Can you work these out from the drawing? Everything is in mm from the part's minimum corner. Coordinates: 2 decimals unless noted, no trailing zeros. Write each loop counter-clockwise with the first axis right and the second up, starting at its lowest first coordinate (ties: lowest second). Pieces come first, ordered by that corner, then holes. Notation, with made-up numbers: M -35.5,66 L 21.5,66 A20 ccw 21.5,86 Z; hole C 26,-18 d5. An arc over 180 degrees is marked long. Write item = value, one per line.
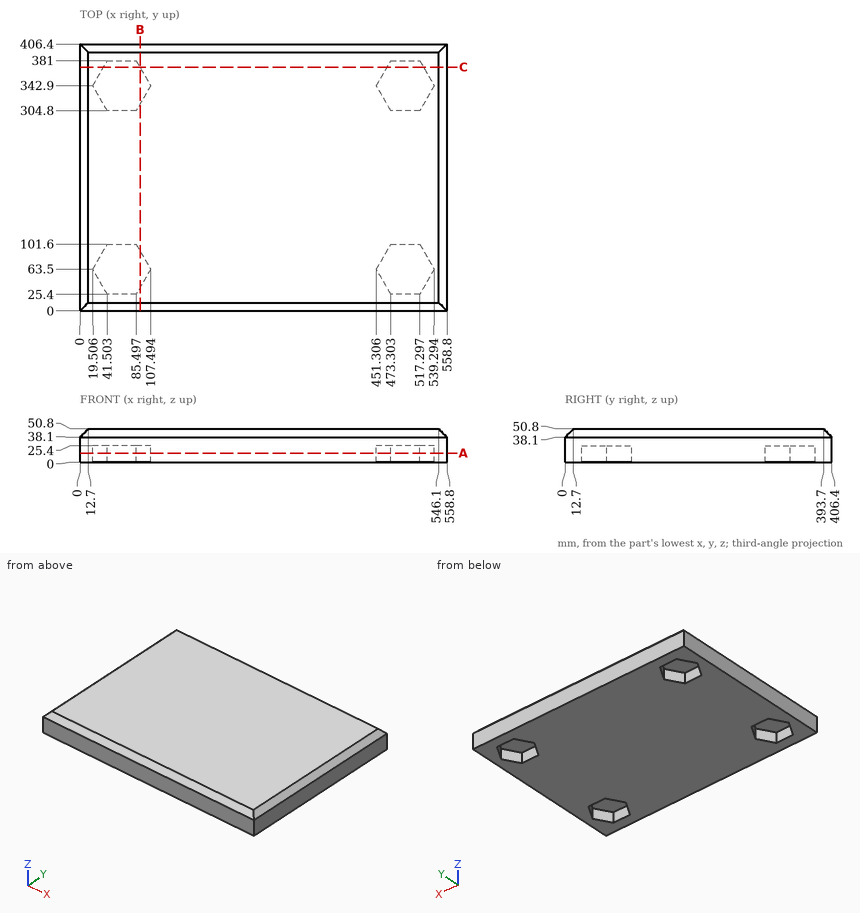
Item 1: If I drill on line 1 along Y through (x, z) = (71, 19); line 2 along X through (y, z) = (354, 6); line 3 along X through (y, z) = (77.5, 10), over which ranges is the centre line in solid material (lowest first)?
Numbers:
line_1 = 0 to 25.4, 101.6 to 304.8, 381 to 406.4
line_2 = 0 to 25.91, 101.09 to 457.71, 532.89 to 558.8
line_3 = 0 to 27.59, 99.41 to 459.39, 531.21 to 558.8
Item 2: Imagine slicing it at A-A (z = 14). Write out the boundary of the cut face in (x, y).
Numbers:
outline = M 0,0 L 558.8,0 L 558.8,406.4 L 0,406.4 Z; hole M 19.51,63.5 L 41.5,25.4 L 85.5,25.4 L 107.49,63.5 L 85.5,101.6 L 41.5,101.6 Z; hole M 19.51,342.9 L 41.5,304.8 L 85.5,304.8 L 107.49,342.9 L 85.5,381 L 41.5,381 Z; hole M 451.31,63.5 L 473.3,25.4 L 517.3,25.4 L 539.29,63.5 L 517.3,101.6 L 473.3,101.6 Z; hole M 451.31,342.9 L 473.3,304.8 L 517.3,304.8 L 539.29,342.9 L 517.3,381 L 473.3,381 Z
Item 3: Imagine slicing it at B-B (x = 91.5). Write out the boundary of the cut face in (y, z), and give its area (3 significant figures).
Numbers:
outline = M 0,0 L 35.8,0 L 35.8,25.4 L 91.2,25.4 L 91.2,0 L 315.2,0 L 315.2,25.4 L 370.6,25.4 L 370.6,0 L 406.4,0 L 406.4,38.1 L 393.7,50.8 L 12.7,50.8 L 0,38.1 Z
area = 17,700 mm²
Item 4: I'm going to push flat-ended pins straight in: P1, Ø4, axis at x = 303, y = 76.5, coming from the -Z side; P2, Ø23, axis at x = 508, y = 343.5, coming from the -Z side; P3, Ø6, axis at y = 166.5, z = 45, coming from the +X side. Where does each tip first touch, or does it pass through?
Numbers:
P1 = 0
P2 = 25.4
P3 = 554.9
Item 5: Imagine slicing it at C-C (y = 371). Write out the boundary of the cut face in (x, z).
Numbers:
outline = M 0,0 L 35.73,0 L 35.73,25.4 L 91.27,25.4 L 91.27,0 L 467.53,0 L 467.53,25.4 L 523.07,25.4 L 523.07,0 L 558.8,0 L 558.8,38.1 L 546.1,50.8 L 12.7,50.8 L 0,38.1 Z
